The listing builds one solid part. Answer for the finished solid, in the listing's coordinates (mm). A direction names the side the tool comes from. Round coordinates to 2 decimals unless told otherwise and drop trailing zeros. Write each loop counter-clockwise with the first axis right and the second up, starting at its lowest first coordinate (ties: lowest second). Pieces come first, ordered by that corner, then holes.
(1) For faces 4 (the face through (0, 1, 5)), 5 (the face through (-23.497, -0.275, 1.972)), determine the directions among +Z, -Z, +X, -X, +Y, -Y from which every point of the face is accessible in a straight line to the end or side of a thin tool.
(2) A cutting plane is placed at A-A, the plane y = 0. Give the vertices of the cut face in (x, z), and give its area (3 significant figures).
(3) A cutting plane is placed at B-B, the plane z = 82.5. Give the vertices of the cut face in (x, y).
(4) The mould has two halves that part along X. Classify faces 1 (the face through (-19.5, -3.52, 52.1)), 2 (the face through (-22.671, -0.257, 4.826)), 3 (the face through (0, 0, 0)): +X half, -X half, draft (parallel to the pull), parting line (faces both ways), or undercut.
(5) Each of these flat-tipped pins is pushed along its axis until it touches: pin 1 Ø2 at (y, z) = (0.5, 86.5) entering from +X; pin 2 Ø3 at (x, z) = (12, 38) entering from -Y; pin 3 Ø10 at (x, z) = (-11.5, 29) entering from +Y. Where does it stop, or does it pass through?
(6) Find the intervals of material crossed by probe 1 along X at (y, z) = (-3, 95.5); probe 2 along X at (y, z) = (-3.25, 47); probe 3 along Y at (x, z) = (11.5, 45), in increasing order.
from build123d import *

# Parameters (mm, degrees)
PAD_DEPTH       = 5
SKETCH001_R     = 9.2
PAD001_DEPTH    = 95
FILLET_R        = 1.5
CHAMFER_SIZE    = 1
CHAMFER001_SIZE = 1


with BuildPart() as part:
    # Sketch → Pad (new body)
    with BuildSketch(Plane.XY):
        with BuildLine():
            ThreePointArc((11, -12.5), (23.5, 0), (11, 12.5))
            Line((11, 12.5), (0, 12.5))
            Line((0, 12.5), (0, -12.5))
            Line((0, -12.5), (11, -12.5))
        make_face()
    pad = extrude(amount=PAD_DEPTH)

    # Mirrored: Pad across Sketch V_Axis
    add(pad.mirror(Plane(origin=(0, 0, 0), x_dir=(0, 0, 1), z_dir=(1, 0, 0))))

    # Sketch001 (on Face5 of Mirrored) → Pad001 (join)
    with BuildSketch(Plane.XY.offset(5)):
        with Locations((11, 0)):
            Circle(SKETCH001_R)
    pad001 = extrude(amount=PAD001_DEPTH)

    # Mirrored001: Pad001 across Sketch001 V_Axis
    add(pad001.mirror(Plane(origin=(0, 0, 5), x_dir=(0, 0, 1), z_dir=(1, 0, 0))))

    # Fillet
    fillet_edges = [part.edges().sort_by_distance(p)[0] for p in [
        (-1.8, 0, 5),
        (1.8, 0, 5),
    ]]
    fillet(fillet_edges, radius=FILLET_R)

    # Chamfer
    chamfer_edges = [part.edges().sort_by_distance(p)[0] for p in [
        (-23.5, 0, 5),
        (0, -12.5, 5),
        (23.5, 0, 5),
        (0, 12.5, 5),
    ]]
    chamfer(chamfer_edges, length=CHAMFER_SIZE)

    # Chamfer001
    chamfer001_edges = [part.edges().sort_by_distance(p)[0] for p in [
        (-1.8, 0, 100),
        (1.8, 0, 100),
    ]]
    chamfer(chamfer001_edges, length=CHAMFER001_SIZE)


solid = part.part
Solutions:
1. face 4: +Z
1. face 5: +Z, -Z, -X
2. outline: (-23.5, 0) - (23.5, 0) - (23.5, 4) - (22.5, 5) - (21.7, 5) arc R1.5 cw to (20.2, 6.5) - (20.2, 99) - (19.2, 100) - (2.8, 100) - (1.8, 99) - (1.8, 6.5) arc R1.5 cw to (0.3, 5) - (-0.3, 5) arc R1.5 cw to (-1.8, 6.5) - (-1.8, 99) - (-2.8, 100) - (-19.2, 100) - (-20.2, 99) - (-20.2, 6.5) arc R1.5 cw to (-21.7, 5) - (-22.5, 5) - (-23.5, 4) - close
2. area: 3,730 mm2
3. outline: circle Ø18.4 at (-11, 0); circle Ø18.4 at (11, 0)
4. face 1: undercut
4. face 2: -X half
4. face 3: draft
5. pin 1: stops at x = 20.2
5. pin 2: stops at y = -9.2
5. pin 3: stops at y = 9.2
6. probe 1: x = -19.7 to -2.3, 2.3 to 19.7
6. probe 2: x = -19.61 to -2.39, 2.39 to 19.61
6. probe 3: y = -9.19 to 9.19
